Input: part model. Units: mm. Frame: model coordinates. Give positions to 0.01 mm unless a question says otherwise; leave off trailing zeros. Loops run counter-clockwise (first coordinate to the right, second up) from the corner with the lowest first, then second, coordinate; pieces in that order, holes last.
from build123d import *

# Parameters (mm, degrees)
F0_R     = 11.1125
F1_DEPTH = 57.15
F3_R     = 7.14375
F4_DEPTH = 114.3
F5_R     = 15.950796
F6_DEPTH = 26.19375
F7_R     = 2.38125
F8_DEPTH = 31.75


with BuildPart() as f1:
    # F0 (on Right) → F1 (new body, symmetric)
    with BuildSketch(Plane.YZ):
        Circle(F0_R)
    extrude(amount=F1_DEPTH, both=True)

    # F3 (on face) → F4 (cut)
    with BuildSketch(Plane.YZ.offset(57.15)):
        Circle(F3_R)
    extrude(amount=-F4_DEPTH, mode=Mode.SUBTRACT)

    # F5 (on Top) → F6 (join, symmetric)
    with BuildSketch(Plane.XY):
        with Locations((-0.234567, -26.506469)):
            Circle(F5_R)
    extrude(amount=F6_DEPTH, both=True)

    # F7 (on face) → F8 (join)
    with BuildSketch(Plane.XY.offset(26.19375)):
        with Locations((-0.234567, -26.506469)):
            Circle(F7_R)
    extrude(amount=F8_DEPTH)


solid = f1.part
(1) Cut plane A-A (y = 0). Return the cut outline in (x, z), and give its area (3 significant figures).
Values follow:
outline: (-57.15, -11.11) - (57.15, -11.11) - (57.15, -7.14) - (-57.15, -7.14) - close; (-57.15, 7.14) - (57.15, 7.14) - (57.15, 11.11) - (-57.15, 11.11) - close
area: 907 mm2
(2) Cut plane C-C (z = 0). Return the cut outline in (x, y), and give its area (3 significant figures).
Values follow:
outline: (-57.15, -11.11) - (-4.41, -11.11) arc R15.95 ccw (long way) to (3.94, -11.11) - (57.15, -11.11) - (57.15, -7.14) - (-57.15, -7.14) - close; (-57.15, 7.14) - (57.15, 7.14) - (57.15, 11.11) - (-57.15, 11.11) - close
area: 1,700 mm2
(3) Cut plane B-B (x = 31.5). Return the cut outline in (y, z) (1 decimal).
Values follow:
outline: circle Ø22.2 at (0, 0); hole circle Ø14.3 at (0, 0)
(4) Mould query, pull axis Y, two halves, no side actions, for faces 1 (the cylindrical face through (0.8, 10.265, -4.256)), 2 (the flat face through (0, -26, -26.194)), 3 (the cylindrical face through (-0.75, -28.83, 41.85)). Classes: +Y half, -Y half, draft (parallel to the pull), parting line (faces both ways), or undercut.
Values follow:
face 1: undercut
face 2: draft
face 3: parting line
(5) Pin query (flat end, axial travel): pin 1 Ø10 at (y, z) = (-33.5, 36) entering from +X; pin 2 Ø5 at (x, z) = (16, 6.5) entering from -Y; pin 3 Ø16 at (x, y) = (1.5, -22.5) entering from +Z; pin 4 Ø3 at (y, z) = (-36.5, 23.5) entering from -X. Return the tip coordinate at first contact, or that it passes through.
Values follow:
pin 1: stops at x = 1.07
pin 2: stops at y = -34.62
pin 3: stops at z = 57.94
pin 4: stops at x = -13.74
(6) Ray query, probe 1 along Y at (x, z) = (-1, -5); probe 2 along Y at (x, z) = (26, -0.5); probe 3 along Z at (x, y) = (-16.5, 0). Return the intervals inside material, ascending.
Values follow:
probe 1: y = -42.44 to -10.57, -9.92 to -5.1, 5.1 to 9.92
probe 2: y = -11.1 to -7.13, 7.13 to 11.1
probe 3: z = -11.11 to -7.14, 7.14 to 11.11
(7) Cut plane D-D (x = -4). Return the cut outline in (y, z) (1 decimal), and give its area (3 significant figures).
Values follow:
outline: (-42, -26.2) - (-11, -26.2) - (-11, -1.5) arc R11.1 ccw (long way) to (-11, 1.5) - (-11, 26.2) - (-42, 26.2) - close; hole circle Ø14.3 at (0, 0)
area: 1,850 mm2
